Geometry: final body of the model. Coordinates: model frame, mm. Face numbers are marked on the shaded views. A direction names the side the tool comes from. Give positions to 0.01 mm unless a question says otherwise; leave off trailing zeros. Loops run counter-clockwise (first coordinate to the right, second up) from the corner with the lowest first, then second, coordinate; pieces in that order, holes last.
1. Access query for the marked faces 1, 2 and 3. Directions: +Z, -Z, +X, -X, +Y, -Y. A direction counts if a zero-diameter tool reaches every point of the face in a straight line with its end or side. Return the directions, or none.
2. Section C-C, the plane x = -14. Output: boundary loops of the cut face in (y, z), then the cut area to 3 significant figures.
3. Material intervals for line 1 along Y through (x, z) = (-28.8, 0); line 2 along Y through (x, z) = (-26.5, 0); line 3 along X through (y, z) = (-22, -4.5), sorted ascending.
4. First-contact query: P1, Ø1, axis at y = 28.5, z = 13.5, coming from the +X side; P2, Ø1.5, axis at x = -10, y = -20, coming from the -Z side; P3, Ø5, axis at x = -22.5, y = -22.5, coming from the +Z side. Flat tips, straight axial feed; report the tip coordinate or a pass-through.
5. Draft query along Z for the marked faces 4, 5 and 6. Return one class per face: +Z half, -Z half, draft (parallel to the pull), parting line (faces both ways), or undercut.
6. Section D-D, the plane z = -18. Output: boundary loops of the cut face in (x, y).
from build123d import *

# Parameters (mm, degrees)
FILLET1_R = 1


with BuildPart() as part:
    # Sketch1 → Revolve1 (revolve)
    with BuildSketch(Plane.XY, mode=Mode.PRIVATE) as revolve1_sk:
        Polygon((0, 7.5), (0, 40), (-2.5, 40), (-2.5, 35), (-27.5, 35), (-27.5, 40), (-30, 40), (-30, 30), (-25, 30), (-25, 10), (-30, 10), (-30, 5), (-27.5, 5), (-27.5, 0), (27.5, 0), (27.5, 7.5), align=None)
    revolve(revolve1_sk.sketch.rotate(Axis((-27.5, 0, 0), (1, 0, 0)), 90), axis=Axis((-27.5, 0, 0), (1, 0, 0)))

    # Fillet1
    fillet1_edges = [part.edges().sort_by_distance(p)[0] for p in [
        (-30, 0, -10),
    ]]
    fillet(fillet1_edges, radius=FILLET1_R)


solid = part.part
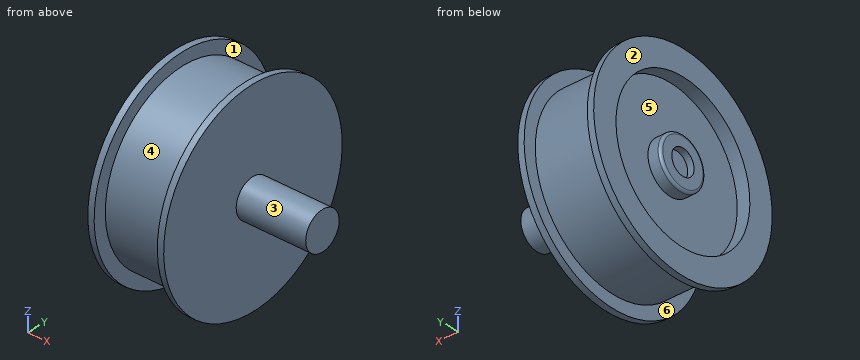
Answers below:
1. face 1: none
1. face 2: +Z, -Z, -X, +Y, -Y
1. face 3: +X
2. outline: circle Ø70 at (0, 0)
2. area: 3,850 mm2
3. line 1: y = -40 to -30, -10 to -5, 5 to 10, 30 to 40
3. line 2: y = -35 to -30, -10 to 10, 30 to 35
3. line 3: x = -25 to 0
4. P1: stops at x = 0
4. P2: stops at z = -29.23
4. P3: stops at z = 28.72
5. face 4: parting line
5. face 5: undercut
5. face 6: draft
6. outline: (-30, -35.72) - (-27.5, -35.72) - (-27.5, -30.02) - (-2.5, -30.02) - (-2.5, -35.72) - (0, -35.72) - (0, 35.72) - (-2.5, 35.72) - (-2.5, 30.02) - (-27.5, 30.02) - (-27.5, 35.72) - (-30, 35.72) - (-30, 24) - (-25, 24) - (-25, -24) - (-30, -24) - close
